The listing builds one solid part. Answer for the finished solid, in the listing's coordinates (mm). A direction names the side the tool comes from. Coordinates: 2 decimals unless noted, no trailing zeros. Order: outer loops, then holes, each group sorted by start corner. A loop starts at its lowest first (then second) coordinate and runs counter-clockwise, first axis right, second up. Notation, with made-up numbers: (10.5, -17.75) - (35.5, -17.75) arc R10 cw to (35.5, -6.75) - close; hole circle Ø4 at (88.25, -8.75). An arc over 180 degrees is marked (long way). Use a Markdown table: item, result. Add a question column.
Item 1: Find the intervals of material crossed by line 1 along X through (y, z) = (-90, -131.5); line 2 along X through (y, z) = (236, 216); line 3 along Z through (x, y) = (-271, 55), in increasing order.
Item 2: For faces 5 (the flat face through (-35, -112, -173)), 6 (the flat face through (-870, -39, 9)), 7 (the flat face through (-35, 53, 32)), 8 (the flat face through (17, 226.771, 272)), determine the directions among +Z, -Z, +X, -X, +Y, -Y from which every point of the face is accessible in a straight line to the end or side of a thin tool.
Item 3: The part is cut by section B-B, the plane z = 477. Give the vertices of the cut face in (x, y), then the cut area to 3 significant figures.
Item 4: The part is cut by section A-A, the plane x = -399.5. Give the vertices of the cut face in (y, z), then the cut area to 3 significant figures.
Item 5: The mould has two halves that part along X. Classify faces 1 (the flat face through (-870, 133, 138)), 2 (the flat face through (0, 133, 138)), 3 (the flat face through (-870, 272, 450)), 4 (the flat face through (-887, 226.771, 272)): released by +X, released by -X, zero draft, split by the parting line, or undercut.
Item 6: The part is cut by section D-D, the plane y = -206. Give the vertices of the cut face in (x, z).
Item 7: The part is cut by section C-C, the plane z = 154. Give the vertices of the cut face in (x, y), then the cut area to 3 significant figures.
Item 8: Flat-ended cylindrical pins translate along their axes: P1, Ø3, axis at x = -604, y = 168.5, coming from the -Z side; P2, Ø6, axis at y = 197, z = 133.5, coming from the +X side; P3, Ø5, axis at x = -494, y = 64.5, coming from the +Z side. Find the tip coordinate at first contact, or state that the pin passes through.
from build123d import *

# Parameters (mm, degrees)
F0_W      = 90
F0_H      = 800
F1_DEPTH  = 35
F3_DEPTH  = 35
F5_W      = 180
F5_H      = 20
F6_DEPTH  = 800
F9_DEPTH  = 35
F10_W     = 90
F10_H     = 800
F11_DEPTH = 35
F12_W     = 35
F12_H     = 90
F13_DEPTH = 275
F4_W      = 35
F4_H      = 90
F14_DEPTH = 275
F15_DEPTH = 15
F16_DEPTH = 15
F17_DEPTH = 15
F18_DEPTH = 15
F19_DEPTH = 15
F20_DEPTH = 15


with BuildPart() as f1:
    # F0 (on Right) → F1 (new body)
    with BuildSketch(Plane.YZ):
        with Locations((271.7706648815, 130.7955920696)):
            Rectangle(F0_W, F0_H)
    extrude(amount=F1_DEPTH)

    # F2 (on face) → F3 (join)
    with BuildSketch(Plane(origin=(0, 0, 0), x_dir=(0, -1, 0), z_dir=(-1, 0, 0))):
        Polygon((248.9147600678, -269.2044079304), (-316.7706648815, 430.7955920696), (-316.7706648815, 287.6064688794), (-84.349539787, 0), (133.2004743535, -269.2044079304), align=None)
    extrude(amount=F3_DEPTH)

    # F5 (on face) → F6 (join)
    with BuildSketch(Plane(origin=(-35, 0, 0), x_dir=(0, -1, 0), z_dir=(-1, 0, 0))):
        with Locations((29.4332100823, -69.2044079304)):
            Rectangle(F5_W, F5_H)
        with Locations((-293.8156041744, 330.7955920696)):
            Rectangle(F5_W, F5_H)
        with Locations((-132.1911970461, 130.7955920696)):
            Rectangle(F5_W, F5_H)
    extrude(amount=F6_DEPTH)

    # F8 (on face) → F9 (join)
    with BuildSketch(Plane(origin=(-835, 0, 0), x_dir=(0, -1, 0), z_dir=(-1, 0, 0))):
        Polygon((-316.7706648815, 430.7955920696), (-316.7706648815, 287.6064688794), (133.2004743535, -269.2044079304), (248.9147600678, -269.2044079304), align=None)
    extrude(amount=F9_DEPTH)

    # F10 (on face) → F11 (join)
    with BuildSketch(Plane(origin=(-870, 0, 0), x_dir=(0, -1, 0), z_dir=(-1, 0, 0))):
        with Locations((-271.7706648815, 130.7955920696)):
            Rectangle(F10_W, F10_H)
    extrude(amount=F11_DEPTH)

    # F12 (on face) → F13 (join)
    with BuildSketch(Plane.XZ.offset(-226.7706648815)):
        with Locations((-887.5, -24.2044079304)):
            Rectangle(F12_W, F12_H)
    extrude(amount=F13_DEPTH)

    # F4 (on face) → F14 (join)
    with BuildSketch(Plane.XZ.offset(-226.7706648815)):
        with Locations((17.5, -24.2044079304)):
            Rectangle(F4_W, F4_H)
    extrude(amount=F14_DEPTH)

    # F5 (on face) → F15 (join)
    with BuildSketch(Plane(origin=(-35, 0, 0), x_dir=(0, -1, 0), z_dir=(-1, 0, 0))):
        with Locations((29.4332100823, -69.2044079304)):
            Rectangle(F5_W, F5_H)
        with Locations((-293.8156041744, 330.7955920696)):
            Rectangle(F5_W, F5_H)
        with Locations((-132.1911970461, 130.7955920696)):
            Rectangle(F5_W, F5_H)
    extrude(amount=-F15_DEPTH)

    # F16 (add): a face of the model
    f16_faces = [f1.faces().sort_by_distance(p)[0] for p in [
        (-835, 58.6012499561, 131.633644551),
    ]]
    extrude(f16_faces, amount=F16_DEPTH)

    # F17 (add): a face of the model
    f17_faces = [f1.faces().sort_by_distance(p)[0] for p in [
        (-835, 205.781144136, 129.9575395882),
    ]]
    extrude(f17_faces, amount=F17_DEPTH)

    # F18 (add): a face of the model
    f18_faces = [f1.faces().sort_by_distance(p)[0] for p in [
        (-835, 220.2256570845, 331.633644551),
    ]]
    extrude(f18_faces, amount=F18_DEPTH)

    # F19 (add): a face of the model
    f19_faces = [f1.faces().sort_by_distance(p)[0] for p in [
        (-835, 350.293134528, 330.7955920696),
    ]]
    extrude(f19_faces, amount=F19_DEPTH)

    # F20 (add): faces of the model
    f20_faces = [f1.faces().sort_by_distance(p)[0] for p in [
        (-835, -103.0231571722, -68.366355449),
        (-835, 44.1567370077, -70.0424604118),
    ]]
    extrude(f20_faces, amount=F20_DEPTH)


solid = f1.part
Solution:
| question | item | result |
|---|---|---|
| 1 | line 1 | x = -870 to -835, -35 to 0 |
| 1 | line 2 | x = -905 to -835, -35 to 35 |
| 1 | line 3 | z = -79.2 to -59.2, 120.8 to 140.8 |
| 2 | face 5 | -Z, +Y, -Y |
| 2 | face 6 | +Z, -Y |
| 2 | face 7 | +Y, -Y |
| 2 | face 8 | +Z, +X, -Y |
| 3 | outline | (-905, 226.77) - (-870, 226.77) - (-870, 316.77) - (-905, 316.77) - close; (0, 226.77) - (35, 226.77) - (35, 316.77) - (0, 316.77) - close |
| 3 | area | 6,300 mm2 |
| 4 | outline | (-119.43, -79.2) - (60.57, -79.2) - (60.57, -59.2) - (-119.43, -59.2) - close; (42.19, 120.8) - (222.19, 120.8) - (222.19, 140.8) - (42.19, 140.8) - close; (203.82, 320.8) - (383.82, 320.8) - (383.82, 340.8) - (203.82, 340.8) - close |
| 4 | area | 10,800 mm2 |
| 5 | face 1 | released by -X |
| 5 | face 2 | released by +X |
| 5 | face 3 | undercut |
| 5 | face 4 | zero draft |
| 6 | outline | (-870, -269.2) - (-835, -269.2) - (-835, -216.1) - (-870, -216.1) - close; (-35, -269.2) - (0, -269.2) - (0, -216.1) - (-35, -216.1) - close |
| 7 | outline | (-905, 226.77) - (-870, 226.77) - (-870, 316.77) - (-905, 316.77) - close; (-870, 93.09) - (-835, 93.09) - (-835, 208.8) - (-870, 208.8) - close; (-35, 93.09) - (0, 93.09) - (0, 208.8) - (-35, 208.8) - close; (0, 226.77) - (35, 226.77) - (35, 316.77) - (0, 316.77) - close |
| 7 | area | 14,400 mm2 |
| 8 | P1 | stops at z = 120.8 |
| 8 | P2 | stops at x = -20 |
| 8 | P3 | stops at z = 140.8 |
